from build123d import *

# Parameters (mm, degrees)
SKETCH_W        = 130
SKETCH_H        = 300
PAD_DEPTH       = 15
SKETCH001_R     = 2.1
SKETCH001_R_2   = 1.2
POCKET_DEPTH    = 15.001
SKETCH002_R     = 4
POCKET001_DEPTH = 6


with BuildPart() as part:
    # Sketch → Pad (new body)
    with BuildSketch(Plane.XZ):
        with Locations((65, 150)):
            Rectangle(SKETCH_W, SKETCH_H)
    extrude(amount=PAD_DEPTH)

    # Sketch001 (on Face6 of Pad) → Pocket (cut, through all)
    with BuildSketch(Plane.XZ.offset(15)):
        with Locations((15, 280)):
            Circle(SKETCH001_R)
        with Locations((45, 280)):
            Circle(SKETCH001_R)
        with Locations((15, 250)):
            Circle(SKETCH001_R)
        with Locations((45, 250)):
            Circle(SKETCH001_R)
        with Locations((85, 280)):
            Circle(SKETCH001_R)
        with Locations((115, 280)):
            Circle(SKETCH001_R)
        with Locations((85, 250)):
            Circle(SKETCH001_R)
        with Locations((115, 250)):
            Circle(SKETCH001_R)
        with Locations((15, 90)):
            Circle(SKETCH001_R)
        with Locations((45, 90)):
            Circle(SKETCH001_R)
        with Locations((15, 60)):
            Circle(SKETCH001_R)
        with Locations((45, 60)):
            Circle(SKETCH001_R)
        with Locations((85, 90)):
            Circle(SKETCH001_R)
        with Locations((115, 90)):
            Circle(SKETCH001_R)
        with Locations((85, 60)):
            Circle(SKETCH001_R)
        with Locations((115, 60)):
            Circle(SKETCH001_R)
        with Locations((35, 235)):
            Circle(SKETCH001_R_2)
        with Locations((95, 235)):
            Circle(SKETCH001_R_2)
        with Locations((35, 210)):
            Circle(SKETCH001_R_2)
        with Locations((95, 210)):
            Circle(SKETCH001_R_2)
        with Locations((35, 185)):
            Circle(SKETCH001_R_2)
        with Locations((95, 185)):
            Circle(SKETCH001_R_2)
        with Locations((35, 160)):
            Circle(SKETCH001_R_2)
        with Locations((95, 160)):
            Circle(SKETCH001_R_2)
        with Locations((35, 135)):
            Circle(SKETCH001_R_2)
        with Locations((95, 135)):
            Circle(SKETCH001_R_2)
        with Locations((35, 110)):
            Circle(SKETCH001_R_2)
        with Locations((95, 110)):
            Circle(SKETCH001_R_2)
        with Locations((35, 85)):
            Circle(SKETCH001_R_2)
        with Locations((95, 85)):
            Circle(SKETCH001_R_2)
        with Locations((35, 60)):
            Circle(SKETCH001_R_2)
        with Locations((95, 60)):
            Circle(SKETCH001_R_2)
        with Locations((35, 35)):
            Circle(SKETCH001_R_2)
        with Locations((95, 35)):
            Circle(SKETCH001_R_2)
        with Locations((35, 10)):
            Circle(SKETCH001_R_2)
        with Locations((95, 10)):
            Circle(SKETCH001_R_2)
    extrude(amount=-POCKET_DEPTH, mode=Mode.SUBTRACT)

    # Sketch002 (on Face5 of Pocket) → Pocket001 (cut)
    with BuildSketch(Plane.XZ.offset(15)):
        with Locations((15, 280.000031)):
            Circle(SKETCH002_R)
        with Locations((45, 280.000031)):
            Circle(SKETCH002_R)
        with Locations((95, 185)):
            Circle(SKETCH002_R)
        with Locations((36.2, 10)):
            Circle(SKETCH002_R)
        with Locations((35, 235)):
            Circle(SKETCH002_R)
        with Locations((85, 60)):
            Circle(SKETCH002_R)
        with Locations((17.1, 60)):
            Circle(SKETCH002_R)
        with Locations((95, 160)):
            Circle(SKETCH002_R)
        with Locations((35, 110)):
            Circle(SKETCH002_R)
        with Locations((35, 185)):
            Circle(SKETCH002_R)
        with Locations((95, 35)):
            Circle(SKETCH002_R)
        with Locations((85, 280)):
            Circle(SKETCH002_R)
        with Locations((95, 10)):
            Circle(SKETCH002_R)
        with Locations((35, 160)):
            Circle(SKETCH002_R)
        with Locations((35, 35)):
            Circle(SKETCH002_R)
        with Locations((95, 110)):
            Circle(SKETCH002_R)
    extrude(amount=-POCKET001_DEPTH, mode=Mode.SUBTRACT)


solid = part.part
Source: CAD feature listing. Evaluate the final solid. Frame: model axes, mm. A direction names the side the tool comes from. Round coordinates to 2 decimals unless told otherwise and drop trailing zeros. Return JSON: item names as keys, results as strings. Group by question number.
1. Material intervals for line 1 along Z through (x, y) = (45, -6.5); line 2 along Z through (x, y) = (45, -12.5); line 3 along X through (y, z) = (-12, 33), sorted ascending. Write a range as from..to.
2. Mould query, pull axis Z, two halves, no side actions, for faces 3 (the face through (36, -9, 161)), 4 (the face through (34.479, -12.042, 163.966)), 5 (the face through (64, -15, 152)). Classes: released by +Z, released by -Z, zero draft, split by the parting line, or undercut.
3. Reachability of faces 1 (the face through (64, 0, 152)), 2 (the face through (36, -9, 186)) from +Z, -Z, +X, -X, +Y, -Y: full face, straight path, thin tool, end or side. Return the list, or none.
4. Pin query (flat end, axial travel): pin 1 (4 mm diameter, centred on x = 95, z = 186.5, fed in from -Y). Return the tip coordinate at first contact, or that it passes through.
Checks:
{
 "1": {"line 1": "z = 0..57.9, 62.1..87.9, 92.1..247.9, 252.1..277.9, 282.1..300", "line 2": "z = 0..57.9, 62.1..87.9, 92.1..247.9, 252.1..276, 284..300", "line 3": "x = 0..31.54, 38.46..91.54, 98.46..130"},
 "2": {"face 3": "undercut", "face 4": "undercut", "face 5": "zero draft"},
 "3": {"face 1": "+Z, -Z, +X, -X, +Y", "face 2": "-Y"},
 "4": {"pin 1": "stops at y = -9"}
}
